```python
from build123d import *

# Parameters (mm, degrees)
SKETCH_1_R          = 16
EXTRUDE_2_DEPTH     = 11
CUT_EXTRUDE_1_DEPTH = 5
SKETCH_4_W          = 5
SKETCH_4_H          = 4
CUT_EXTRUDE_2_DEPTH = 11
SKETCH_5_R          = 2.6
CUT_EXTRUDE_3_DEPTH = 11
SKETCH_6_R          = 5
CUT_EXTRUDE_4_DEPTH = 3
SKETCH_8_R          = 16
SKETCH_8_R_2        = 12
EXTRUDE_5_DEPTH     = 1
EXTRUDE_START       = 2
SKETCH_9_R          = 12
SKETCH_9_R_2        = 5
EXTRUDE_6_DEPTH     = 2
SKETCH_10_R         = 16.1
CUT_EXTRUDE_5_DEPTH = 10
SKETCH_12_W         = 48.107556011
SKETCH_12_H         = 4
EXTRUDE_7_DEPTH     = 5
SKETCH_13_R         = 16.1
EXTRUDE_8_DEPTH     = 5


with BuildPart() as part:
    # 草图1 → 凸台-拉伸2 (new body)
    with BuildSketch(Plane(origin=(0, 0, 0), x_dir=(1, 0, 0), z_dir=(0, 1, 0))):
        with BuildLine():
            Line((50, 14), (-3.107556011, 14))
            ThreePointArc((-3.107556011, 14), (-36.723082923, 0), (-3.107556011, -14))
            Line((-3.107556011, -14), (50, -14))
            Line((50, -14), (50, -10))
            Line((50, -10), (50, 10))
            Line((50, 10), (50, 14))
        make_face()
        with Locations(Location((-17, 0, 0), (0, 0, 270))):
            Circle(SKETCH_1_R, mode=Mode.SUBTRACT)
    extrude(amount=EXTRUDE_2_DEPTH)

    # 草图3 → 切除-拉伸1 (cut)
    with BuildSketch(Plane(origin=(0, 11, 0), x_dir=(1, 0, 0), z_dir=(0, 1, 0))):
        Polygon((0, 0), (0, 10), (45, 10), (45, -10), (0, -10), align=None)
    extrude(amount=-CUT_EXTRUDE_1_DEPTH, mode=Mode.SUBTRACT)

    # 草图4 → 切除-拉伸2 (cut)
    with BuildSketch(Plane(origin=(0, 11, 0), x_dir=(1, 0, 0), z_dir=(0, 1, 0))):
        with Locations((47.5, 12)):
            Rectangle(SKETCH_4_W, SKETCH_4_H)
        Polygon((45, -14), (50, -14), (50, 10), (45, 10), (45, -10), align=None)
    extrude(amount=-CUT_EXTRUDE_2_DEPTH, mode=Mode.SUBTRACT)

    # 草图5 → 切除-拉伸3 (cut)
    with BuildSketch(Plane(origin=(0, 6, 0), x_dir=(1, 0, 0), z_dir=(0, 1, 0))):
        with Locations(Location((15, 0, 0), (0, 0, 270))):
            Circle(SKETCH_5_R)
        with Locations(Location((30, 0, 0), (0, 0, 270))):
            Circle(SKETCH_5_R)
    extrude(amount=-CUT_EXTRUDE_3_DEPTH, mode=Mode.SUBTRACT)

    # 草图6 → 切除-拉伸4 (cut)
    with BuildSketch(Plane.XZ):
        with Locations(Location((15, 0, 0), (0, 0, 270))):
            Circle(SKETCH_6_R)
        with Locations(Location((30, 0, 0), (0, 0, 270))):
            Circle(SKETCH_6_R)
    extrude(amount=-CUT_EXTRUDE_4_DEPTH, mode=Mode.SUBTRACT)

    # 草图8 → 凸台-拉伸5 (add)
    with BuildSketch(Plane(origin=(0, 0, 0), x_dir=(-1, 0, 0), z_dir=(0, -1, 0))):
        with Locations(Location((17, 0, 0), (0, 0, 90))):
            Circle(SKETCH_8_R)
        with Locations(Location((17, 0, 0), (0, 0, 90))):
            Circle(SKETCH_8_R_2, mode=Mode.SUBTRACT)
    extrude(amount=-EXTRUDE_5_DEPTH)

    # 草图9 → 凸台-拉伸6 (add)
    with BuildSketch(Plane.XZ.offset(EXTRUDE_START)):
        with BuildLine():
            Line((-3.107556011, 14), (45, 14))
            Line((45, 14), (45, -14))
            Line((45, -14), (-3.107556011, -14))
            ThreePointArc((-3.107556011, -14), (-36.723082923, 0), (-3.107556011, 14))
        make_face()
        with Locations(Location((-17, 0, 0), (0, 0, 270))):
            Circle(SKETCH_9_R, mode=Mode.SUBTRACT)
        with Locations(Location((15, 0, 0), (0, 0, 270))):
            Circle(SKETCH_9_R_2, mode=Mode.SUBTRACT)
        with Locations(Location((30, 0, 0), (0, 0, 270))):
            Circle(SKETCH_9_R_2, mode=Mode.SUBTRACT)
    extrude(amount=-EXTRUDE_6_DEPTH)

    # 草图10 → 切除-拉伸5 (cut)
    with BuildSketch(Plane(origin=(0, 11, 0), x_dir=(1, 0, 0), z_dir=(0, 1, 0))):
        with Locations(Location((-17, 0, 0), (0, 0, 270))):
            Circle(SKETCH_10_R)
    extrude(amount=-CUT_EXTRUDE_5_DEPTH, mode=Mode.SUBTRACT)

    # 草图12 → 凸台-拉伸7 (add)
    with BuildSketch(Plane(origin=(0, 11, 0), x_dir=(1, 0, 0), z_dir=(0, 1, 0))):
        with Locations((20.946221995, 12)):
            Rectangle(SKETCH_12_W, SKETCH_12_H)
        with Locations((20.946221995, -12)):
            Rectangle(SKETCH_12_W, SKETCH_12_H)
    extrude(amount=EXTRUDE_7_DEPTH)

    # 草图13 → 凸台-拉伸8 (add)
    with BuildSketch(Plane(origin=(0, 11, 0), x_dir=(1, 0, 0), z_dir=(0, 1, 0))):
        with BuildLine():
            Line((-3.107556011, 14), (0, 10))
            Line((0, 10), (0, -10))
            ThreePointArc((0, -10), (-36.559799946, -2.532632245), (-3.107556011, 14))
        make_face()
        with Locations(Location((-17, 0, 0), (0, 0, 270))):
            Circle(SKETCH_13_R, mode=Mode.SUBTRACT)
    extrude(amount=EXTRUDE_8_DEPTH)


solid = part.part
```
The model under review builds one solid part; all positions refer to its coordinate system, in mm. A direction names the side the tool comes from. Coordinates: 2 decimals unless noted, no trailing zeros. Write each loop counter-clockwise with the first axis right and the second up, starting at its lowest first coordinate (ties: lowest second). Pieces come first, ordered by that corner, then holes. Notation, with made-up numbers: (-20.75, -12.75) - (-8.75, -12.75) arc R21 ccw to (-8.75, 24.25) - close; hole circle Ø3 at (-3, 25). An arc over 180 degrees is marked (long way). Answer in a Markdown table with one row per item. Add a question column.
Q1. Consider section C-C on z = 0. Give the number of separate pieces and of enclosed holes in the cut face, then the cut area to 3 significant figures.
Q2. Consider section B-B on y = 12.25. Give the boundary of the cut face in (x, z), then the cut area to 3 significant figures.
Q3. Clearance check with flat-ended pins moving along their axes: pin 1 (1 mm diameter, centred on x = 18, z = 2, fed in from +Y); pin 2 (5.5 mm diameter, centred on y = 13.5, z = -1.5, fed in from +X); pin 3 (5 mm diameter, centred on x = 19.5, y = 12.5, fed in from +Z). State where each tip first meets the part, or that it passes through.
Q4. Draft analysis for pull direction X (two halves, no side actions). For faces 6 (the face through (45, 3, 0)), 7 (the face through (25.12, 0.46, 1.08)), 8 (the face through (23, 6, 0)), 9 (the face through (28, 3, -2)), state which applies: +X half, -X half, draft (parallel to the pull), parting line (faces both ways), or undercut.
Q5. Consider section A-A on x = -17. Give the boundary of the cut face in (y, z).
Q6. To check wall thickness, follow line 1 along X through (y, z) = (-0.2, 0); line 2 along X through (y, z) = (5.3, 0); line 3 along Z through (x, y) = (29, 8.5). State the ranges of each line that lie inside material, in increasing order. Write a range as from..to.
Q7. Consider section D-D on z = 6. Give the boundary of the cut face in (x, y).
Q8. For faces 1 (the face through (21, 7, -14)), 2 (the face through (21, 7, 14)), 3 (the face through (-5, 1, -2)), 4 (the face through (13, 3, -2)), 5 (the face through (22, 11, 10)), list the 3-axis set-ups (+Z, -Z, +X, -X, +Y, -Y) from which the entire face can be reached by the end or side of a thin tool; tool diameter is ignored.
Answers below:
| question | item | result |
|---|---|---|
| 1 | separate pieces | 4 |
| 1 | enclosed holes | 0 |
| 1 | area | 335 mm² |
| 2 | outline | (-3.11, -14) - (45, -14) - (45, -10) - (0, -10) - (0, 10) - (45, 10) - (45, 14) - (-3.11, 14) arc R19.72 ccw (long way) to start; hole circle Ø32.2 at (-17, 0) |
| 2 | area | 742 mm² |
| 3 | pin 1 | y = 6 |
| 3 | pin 2 | x = 0 |
| 3 | pin 3 | z = 14 |
| 4 | face 6 | +X half |
| 4 | face 7 | undercut |
| 4 | face 8 | draft |
| 4 | face 9 | undercut |
| 5 | outline | (-2, -19.72) - (16, -19.72) - (16, -16.1) - (1, -16.1) - (1, -12) - (-2, -12) - close; (-2, 12) - (1, 12) - (1, 16.1) - (16, 16.1) - (16, 19.72) - (-2, 19.72) - close |
| 6 | line 1 | -36.72..-29, -5..10, 20..25, 35..45 |
| 6 | line 2 | -36.72..-33.1, -0.9..12.4, 17.6..27.4, 32.6..45 |
| 6 | line 3 | -14..-10, 10..14 |
| 7 | outline | (-35.79, -2) - (-27.39, -2) - (-27.39, 1) - (-31.94, 1) - (-31.94, 16) - (-35.79, 16) - close; (-6.61, -2) - (45, -2) - (45, 6) - (0, 6) - (0, 16) - (-2.06, 16) - (-2.06, 1) - (-6.61, 1) - close |
| 8 | face 1 | -Z, +X, +Y, -Y |
| 8 | face 2 | +Z, +X, +Y, -Y |
| 8 | face 3 | +Y |
| 8 | face 4 | -Y |
| 8 | face 5 | +X, +Y |
